Here's how the part is built. I have some questions about the finished solid (model axes, mm). Give positions to 0.01 mm unless a question says otherwise; leave off trailing zeros. Loops run counter-clockwise (first coordinate to the right, second up) from the corner with the lowest first, then second, coordinate; pieces in that order, holes last.
Q1. Thinking about a two-plate mould opening in X: for faces 1 (the face through (-6.045, -271.622, -1.014)), 2 (the face through (-4, 4, 0)), which applies, pulls with the +X half, pulls with the -X half, needs draft (parallel to the pull), parting line crosses it, or undercut?
Q2. Suppose I cut it at A-A (y = -260). List the corners of the cut face in (x, z) for me.
Q3. I need wall thicknesses on probe 1 along X at (y, z) = (280, -0.6); probe 2 along Y at (x, z) = (240, -1.25); probe 3 along Y at (x, z) = (0, -0.8). Which ranges of each line are inside material? Lowest first, please.
```python
from build123d import *

# Parameters (mm, degrees)
SZKIC1_W                   = 550
SZKIC1_H                   = 580
ODGI_CIE_BAZOWE1_DEPTH     = 2
ZAOKR_GLENIE1_R            = 5
WYTNIJ_WYCI_GNI_CIE2_REACH = 401.661
SZKIC3_R                   = 2.1
WYTNIJ_WYCI_GNI_CIE3_REACH = 401.661
SZKIC4_R                   = 13.1


# Sheet-metal steps are written as plain solids
with BuildPart() as part:
    # Szkic1 → Odgięcie bazowe1 (new body)
    with BuildSketch(Plane.XY):
        Rectangle(SZKIC1_W, SZKIC1_H)
    extrude(amount=-ODGI_CIE_BAZOWE1_DEPTH)

    # Zaokrąglenie1
    zaokr_glenie1_edges = [part.edges().sort_by_distance(p)[0] for p in [
        (275, -290, -1),
        (-275, -290, -1),
    ]]
    fillet(zaokr_glenie1_edges, radius=ZAOKR_GLENIE1_R)

    # Szkic3 → Wytnij-wyciągnięcie2 (cut, up to next)
    with BuildSketch(Plane.XY, mode=Mode.PRIVATE) as wytnij_wyci_gni_cie2_sk1:
        with Locations((0, 280)):
            Circle(SZKIC3_R)
    wytnij_wyci_gni_cie2_tool1 = extrude(wytnij_wyci_gni_cie2_sk1.sketch, amount=-WYTNIJ_WYCI_GNI_CIE2_REACH, mode=Mode.PRIVATE) & part.part
    # Szkic3 → Wytnij-wyciągnięcie2 (cut, up to next)
    with BuildSketch(Plane.XY, mode=Mode.PRIVATE) as wytnij_wyci_gni_cie2_sk2:
        with Locations((120, 280)):
            Circle(SZKIC3_R)
    wytnij_wyci_gni_cie2_tool2 = extrude(wytnij_wyci_gni_cie2_sk2.sketch, amount=-WYTNIJ_WYCI_GNI_CIE2_REACH, mode=Mode.PRIVATE) & part.part
    # Szkic3 → Wytnij-wyciągnięcie2 (cut, up to next)
    with BuildSketch(Plane.XY, mode=Mode.PRIVATE) as wytnij_wyci_gni_cie2_sk3:
        with Locations((240, 280)):
            Circle(SZKIC3_R)
    wytnij_wyci_gni_cie2_tool3 = extrude(wytnij_wyci_gni_cie2_sk3.sketch, amount=-WYTNIJ_WYCI_GNI_CIE2_REACH, mode=Mode.PRIVATE) & part.part
    # Szkic3 → Wytnij-wyciągnięcie2 (cut, up to next)
    with BuildSketch(Plane.XY, mode=Mode.PRIVATE) as wytnij_wyci_gni_cie2_sk4:
        with Locations(Location((-240, 280, 0), (0, 0, 180))):
            Circle(SZKIC3_R)
    wytnij_wyci_gni_cie2_tool4 = extrude(wytnij_wyci_gni_cie2_sk4.sketch, amount=-WYTNIJ_WYCI_GNI_CIE2_REACH, mode=Mode.PRIVATE) & part.part
    # Szkic3 → Wytnij-wyciągnięcie2 (cut, up to next)
    with BuildSketch(Plane.XY, mode=Mode.PRIVATE) as wytnij_wyci_gni_cie2_sk5:
        with Locations(Location((-120, 280, 0), (0, 0, 180))):
            Circle(SZKIC3_R)
    wytnij_wyci_gni_cie2_tool5 = extrude(wytnij_wyci_gni_cie2_sk5.sketch, amount=-WYTNIJ_WYCI_GNI_CIE2_REACH, mode=Mode.PRIVATE) & part.part
    add(wytnij_wyci_gni_cie2_tool1.solids().sort_by_distance((0, 280, 0))[0], mode=Mode.SUBTRACT)
    add(wytnij_wyci_gni_cie2_tool2.solids().sort_by_distance((120, 280, 0))[0], mode=Mode.SUBTRACT)
    add(wytnij_wyci_gni_cie2_tool3.solids().sort_by_distance((240, 280, 0))[0], mode=Mode.SUBTRACT)
    add(wytnij_wyci_gni_cie2_tool4.solids().sort_by_distance((-240, 280, 0))[0], mode=Mode.SUBTRACT)
    add(wytnij_wyci_gni_cie2_tool5.solids().sort_by_distance((-120, 280, 0))[0], mode=Mode.SUBTRACT)

    # Szkic4 → Wytnij-wyciągnięcie3 (cut, up to next)
    with BuildSketch(Plane(origin=(0, 0, -2), x_dir=(-1, 0, 0), z_dir=(0, 0, -1)), mode=Mode.PRIVATE) as wytnij_wyci_gni_cie3_sk1:
        with Locations((0, -260)):
            Circle(SZKIC4_R)
    wytnij_wyci_gni_cie3_tool1 = extrude(wytnij_wyci_gni_cie3_sk1.sketch, amount=-WYTNIJ_WYCI_GNI_CIE3_REACH, mode=Mode.PRIVATE) & part.part
    add(wytnij_wyci_gni_cie3_tool1.solids().sort_by_distance((0, -260, -2))[0], mode=Mode.SUBTRACT)


solid = part.part
```
Solutions:
1. face 1: undercut
1. face 2: needs draft
2. outline: (-275, -2) - (-13.1, -2) - (-13.1, 0) - (-275, 0) - close; (13.1, -2) - (275, -2) - (275, 0) - (13.1, 0) - close
3. probe 1: x = -275 to -242.1, -237.9 to -122.1, -117.9 to -2.1, 2.1 to 117.9, 122.1 to 237.9, 242.1 to 275
3. probe 2: y = -290 to 277.9, 282.1 to 290
3. probe 3: y = -290 to -273.1, -246.9 to 277.9, 282.1 to 290
